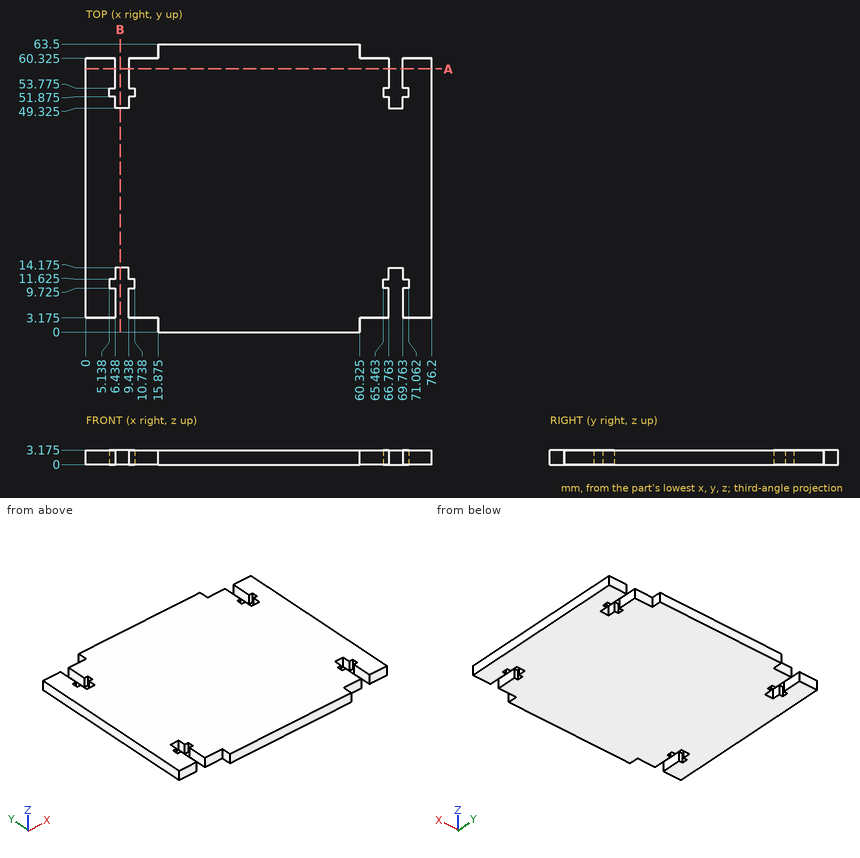
The drawing under review shows one solid part. Ordinate dimensions are in mm from its lowest x, y, z. Round coordinates to 2 decimals unless told otherwise and drop trailing zeros. Write each loop counter-clockwise with the first axis right and the second up, starting at its lowest first coordinate (ties: lowest second). Pieces come first, ordered by that corner, then holes.
(1) We need section B-B on x = 7.5. Give the boundary of the cut face in (y, z) (1 decimal).
(2) Wall thickness on L1, parallel to X at y = 11.5, z = 0.35; L2, parallel to X at y = 55, z = 2.3; L3, parallel to Y at x = 65.5, z = 2.65 (1 decimal): over which ranges is each line inside the solid? List them lowest first.
(3) Insertion check: pin 1 (1 mm diameter, centred on x = 66.5, z = 2.5, fed in from -Y) (1 decimal); pin 2 (1.6 mm diameter, centred on y = 2, z = 2, fed in from -X) (1 decimal); pin 3 (1.4 mm diameter, centred on x = 66, z = 1, fed in from +Y) (1 decimal). Each pin has a flat end and moves straight along its axis. Give the tip position at first contact, or say it passes through.
(4) We need section A-A on y = 58. Give the boundary of the cut face in (x, z) (1 decimal).
Findings below:
1. outline: (14.2, 0) - (49.3, 0) - (49.3, 3.2) - (14.2, 3.2) - close
2. L1: x = 0 to 5.14, 10.74 to 65.46, 71.06 to 76.2
2. L2: x = 0 to 6.44, 9.44 to 66.76, 69.76 to 76.2
2. L3: y = 3.2 to 9.7, 11.6 to 51.9, 53.8 to 60.3
3. pin 1: stops at y = 3.2
3. pin 2: stops at x = 15.9
3. pin 3: stops at y = 60.3
4. outline: (0, 0) - (6.4, 0) - (6.4, 3.2) - (0, 3.2) - close; (9.4, 0) - (66.8, 0) - (66.8, 3.2) - (9.4, 3.2) - close; (69.8, 0) - (76.2, 0) - (76.2, 3.2) - (69.8, 3.2) - close
